Can you work these out from the model? Positions are in its coordinate system, mm. A direction names the side the tool comes from. Coordinates: 2 decimals unless noted, no trailing zeros. Loops run counter-clockwise (first coordinate to the right, second up) from the corner with the lowest first, then second, coordinate; pieces in that order, holes last.
Autodesk Inventor part; units mm, degrees
ref_plane "YZ Plane" through (0, 0, 0) normal (1, 0, 0) x (0, 1, 0)
ref_plane "XZ Plane" through (0, 0, 0) normal (0, 1, 0) x (-1, 0, 0)
ref_plane "XY Plane" through (0, 0, 0) normal (0, 0, 1) x (1, 0, 0)
sketch "Sketch1" plane through (0, 0, 0) normal (0, 0, 1) x (1, 0, 0)
  line L0 (0, 0) -> (23.114, 0)
  line L1 (23.114, 0) -> (23.114, 15.0368)
  line L2 (23.114, 15.0368) -> (0, 15.0368)
  line L3 (0, 15.0368) -> (0, 0)
  dimension "d0" = 15.0368
  dimension "d1" = 23.114
extrude "Extrusion1" add sketch "Sketch1" along normal blind 11.7348
sketch "Sketch2" plane through (0, 0, 11.7348) normal (0, 0, 1) x (1, 0, 0)
  line L0 (23.114, 0) -> (23.114, 3.6138)
  line L1 (23.114, 0) -> (23.114, 15.0368)
  line L2 (0, 0) -> (23.114, 0)
  line L3 (20.3034, 0) -> (23.114, 0)
  line L4 (23.114, 3.6138) -> (20.3034, 0)
extrude "Extrusion2" cut sketch "Sketch2" against normal blind 11.7348
sketch "Sketch3" plane through (0, 0, 11.7348) normal (0, 0, 1) x (1, 0, 0)
  line L0 (-4.6433, 16.5606) -> (27.1067, 16.5606)
  line L1 (27.1067, 16.5606) -> (27.1067, 15.0366)
  line L2 (27.1067, 15.0366) -> (-4.6433, 15.0366)
  line L3 (-4.6433, 15.0366) -> (-4.6433, 16.5606)
  line L4 (23.114, 15.0368) -> (0, 15.0368)
  point P0 (0, 0)
  dimension "d6" = 31.75
  dimension "d7" = 1.524
extrude "Extrusion3" add sketch "Sketch3" against normal blind 11.7348
sketch "Sketch4" plane through (0, 0, 11.7348) normal (0, 0, 1) x (1, 0, 0)
  line L0 (-4.6433, 16.5606) -> (27.1067, 16.5606)
  line L1 (0, 16.5606) -> (23.1157, 16.5606)
  line L2 (23.1157, 16.5606) -> (23.1157, 21.3866)
  line L3 (23.1157, 21.3866) -> (0, 21.3866)
  line L4 (0, 21.3866) -> (0, 16.5606)
  point P0 (0, 0)
  dimension "d10" = 4.826
extrude "Extrusion4" add sketch "Sketch4" against normal up to surface (11.7348 mm away)
sketch "Sketch5" plane through (0, 21.3866, 11.7348) normal (0, 1, 0) x (1, 0, 0)
  circle A0 centre (16.7403, 5.8674) radius 4.8959
  point P0 (0, 11.7348)
  dimension "d14" = 9.7917
extrude "Extrusion5" add sketch "Sketch5" along normal blind 3.9878
sketch "Sketch6" plane through (16.7403, 25.3744, 5.8674) normal (0, 1, 0) x (1, 0, 0)
  circle A0 centre (0, 0) radius 4.8958
  arc A1 (-3.876, 2.991) -> (-5.6698, 0.5745) centre (-4.3859, 1.4955) ccw
  line L0 (-5.6698, 0.5745) -> (-6.3204, 0.5745)
  line L1 (-6.3204, 0.5745) -> (-6.3204, -2.991)
  line L2 (-6.3204, -2.991) -> (-3.876, -2.991)
  line L3 (-3.876, 0) -> (-3.876, 0.5745)
  point P0 (-16.7403, 5.8674)
extrude "Extrusion6" add sketch "Sketch6" against normal blind 3.9878 contours A0 L2 L1 L0 A1
sketch "Sketch7" plane through (0, 25.3744, 11.7348) normal (0, 1, 0) x (1, 0, 0)
  circle A0 centre (16.9713, 5.8977) radius 1.7145
  point P0 (0, 11.7348)
  dimension "d19" = 3.429
extrude "Extrusion7" add sketch "Sketch7" along normal blind 2.9718
sketch "Sketch8" plane through (16.9713, 28.3462, 5.8371) normal (0, 1, 0) x (1, 0, 0)
  circle A0 centre (0, 0) radius 0.41
  point P0 (-16.9713, 5.8371)
extrude "Extrusion8" cut sketch "Sketch8" against normal blind 0.254
Item 1: Suppose I cut it at B-B, the plane y = 20.75. Please give me the cut outline in (x, z).
Results are:
outline: (0, 0) - (23.12, 0) - (23.12, 11.73) - (0, 11.73) - close
Item 2: I need wall thicknesses on line 1 along X through (y, z) = (19, 4.75); line 2 along Y through (x, z) = (15, 2); line 3 along Y through (x, z) = (5, 10.75). Which ranges of each line are inside material? Lowest first, please.
Results are:
line 1: x = 0 to 23.12
line 2: y = 0 to 25.37
line 3: y = 0 to 21.39
Item 3: Suppose I cut it at A-A, the plane x = 12.5. Please give me the cut outline in (y, z).
Results are:
outline: (0, 0) - (21.39, 0) - (21.39, 2.8) - (25.37, 2.8) - (25.37, 8.86) - (21.39, 8.86) - (21.39, 11.73) - (0, 11.73) - close
Item 4: Suppose I cut it at D-D, the plane x = 4. Please give me the cut outline in (y, z).
Results are:
outline: (0, 0) - (21.39, 0) - (21.39, 11.73) - (0, 11.73) - close
Item 5: On a 3-axis mill with a long thin cutter (end or side, diameter ignored), from which of +Z, -Z, +X, -X, +Y, -Y can I reach the whole of each face in a straight line? I mean faces 1 (the face through (-2, 15.037, 6)), 2 (the face through (12, 23, 8.858)), 3 (the face through (21.633, 23.353, 5.697)). Say none if no direction works.
Results are:
face 1: +Z, -Z, -X, -Y
face 2: +Z, -X, +Y
face 3: +Y
Item 6: Suppose I cut it at C-C, the plane z = 3.5. Please give me the cut outline in (x, y).
Results are:
outline: (-4.64, 15.04) - (0, 15.04) - (0, 0) - (20.3, 0) - (23.11, 3.61) - (23.11, 15.04) - (27.11, 15.04) - (27.11, 16.56) - (23.12, 16.56) - (23.12, 21.39) - (21.03, 21.39) - (21.03, 25.37) - (11.04, 25.37) - (11.04, 21.39) - (0, 21.39) - (0, 16.56) - (-4.64, 16.56) - close
Item 7: We'd pull the mould along X, two halves only. Please class faces 4 (the face through (-4.643, 16, 6)), 5 (the face through (11, 11, 0)), 6 (the face through (21.728, 1.832, 5.95)): +X half, -X half, draft (parallel to the pull), parting line (faces both ways), or undercut.
Results are:
face 4: -X half
face 5: draft
face 6: +X half
Item 8: I'm going to push flat-ended pins straight in: P1, Ø3.5, axis at x = -3.5, z = 7, coming from the -Y side; P2, Ø2, axis at y = 22.5, z = 6.5, coming from the +X side; P3, Ø6, axis at x = 11.5, z = 4, coming from the +Y side. Where does each tip first touch, or does it pass through?
Results are:
P1: stops at y = 15.04
P2: stops at x = 21.64
P3: stops at y = 25.37
